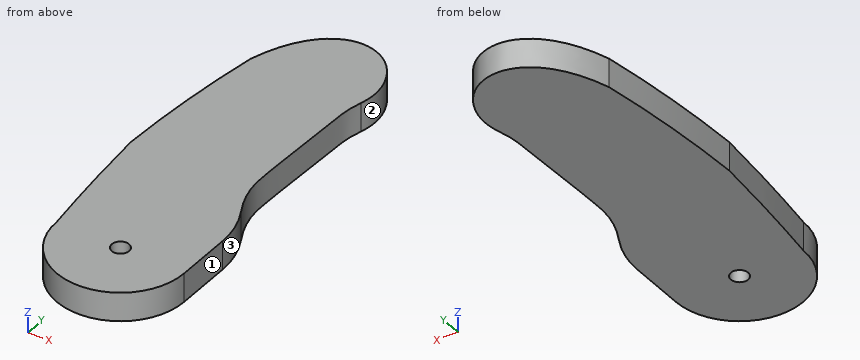
```python
from build123d import *

# Parameters (mm, degrees)
BOSS_EXTRUDE1_DEPTH = 5
SKETCH2_R           = 1.5
CUT_EXTRUDE1_DEPTH  = 15


with BuildPart() as part:
    # Sketch1 → Boss-Extrude1 (new body)
    with BuildSketch(Plane.XY):
        with BuildLine():
            Line((-22.025473837, -12.460288432), (-22.025473837, -22.099692602))
            ThreePointArc((-22.025473837, -22.099692602), (-33.089336525, -33.163555291), (-44.153199213, -22.099692602))
            add(Edge.make_bspline(
                [(-46.60586196, 0), (-45.711257539, -11.089055713), (-44.153199213, -22.099692602)],
                knots=[0, 0, 0, 1, 1, 1], degree=2))
            add(Edge.make_bspline(
                [(-46.60586196, 0), (-46.258692623, 13.374484171), (-44.153199213, 26.582155094)],
                knots=[0, 0, 0, 1, 1, 1], degree=2))
            add(Edge.make_bspline(
                [(-44.153199213, 26.582155094), (-39.900483867, 41.183407978), (-29.408706967, 40.976444126), (-25.777388315, 34.042216579)],
                knots=[0, 0, 0, 0, 0.860338307, 0.860338307, 0.860338307, 0.860338307], degree=3))
            ThreePointArc((-25.777388315, 34.042216579), (-24.684371632, 30.383671766), (-25.042291473, 26.582155094))
            add(Edge.make_bspline(
                [(-25.042291473, 26.582155094), (-25.760015873, 24.141164965), (-25.719709218, 19.504814476), (-26.307467845, 6.668994266), (-26.250257145, -0.88224048), (-23.851756529, -5.287201768)],
                knots=[0.083338388, 0.083338388, 0.083338388, 0.083338388, 0.311519057, 0.73939734, 0.959193523, 0.959193523, 0.959193523, 0.959193523], degree=3))
            ThreePointArc((-23.851756529, -5.287201768), (-22.489212976, -8.759326369), (-22.025473837, -12.460288432))
        make_face()
    extrude(amount=BOSS_EXTRUDE1_DEPTH)

    # Sketch2 → Cut-Extrude1 (cut)
    with BuildSketch(Plane.XY.offset(5)):
        with Locations((-33.089336525, -22.099692602)):
            Circle(SKETCH2_R)
    extrude(amount=-CUT_EXTRUDE1_DEPTH, mode=Mode.SUBTRACT)


solid = part.part
```
Check sheet for the modelled part. Datum: model origin and axes. Units: mm. Face numbers are marked on the shaded views. Coordinates: 2 decimals unless noted, no trailing zeros. Use a Markdown table: item, result.
1. Release check for a two-part mould opening along Y. For the marked faces 1, 2 and 3 record: pulls with the +Y half, pulls with the -Y half, needs draft (parallel to the pull), parting line crosses it, or undercut.
Reported:
| item | result |
|---|---|
| face 1 | needs draft |
| face 2 | undercut |
| face 3 | pulls with the +Y half |
2. Scan lines: line 1 along Y through (x, z) = (-33, 1.85); line 2 along Y through (x, z) = (-42.75, 4.4); line 3 along X through (y, z) = (20.5, 2.45). Record each from-to range of solid material in increasing order.
Reported:
| item | result |
|---|---|
| line 1 | y = -33.16 to -23.6, -20.6 to 38.62 |
| line 2 | y = -27.49 to 30.42 |
| line 3 | x = -45.03 to -25.79 |
3. Go/stop test with flat-tipped pins: pin 1 Ø2 at (y, z) = (9.5, 3) entering from -X; pin 2 Ø3 at (x, z) = (-27.5, 2) entering from +Y. Record where each tip stops, or that it passes through.
Reported:
| item | result |
|---|---|
| pin 1 | stops at x = -46.21 |
| pin 2 | stops at y = 37.54 |
